CAD build for the part. Positions are in the model's coordinates, mm. A direction names the side the tool comes from. Give positions to 0.01 mm unless a question says otherwise; leave off trailing zeros. Order: outer loops, then holes, each group sorted by start corner. A loop starts at its lowest first (then second) coordinate and runs counter-clockwise, first axis right, second up.
```python
from build123d import *

# Parameters (mm, degrees)
SKETCH1_R               = 1.6
BOSS_EXTRUDE1_DEPTH     = 60
CUT_EXTRUDE1_DEPTH      = 165.822631941
SKETCH4_R               = 1.6
CUT_EXTRUDE2_DEPTH      = 165.822632055
CUT_EXTRUDE3_DEPTH      = 31.25
CUT_EXTRUDE3_DEPTH_BACK = 31.25
SKETCH5_W               = 5.6
SKETCH5_H               = 30
SKETCH8_R               = 1.6
CUT_EXTRUDE6_DEPTH      = 5
FILLET1_R               = 2
FILLET2_R               = 2
FILLET3_R               = 2
FILLET4_R               = 2
SKETCH9_W               = 7
SKETCH9_H               = 5.6
CUT_EXTRUDE7_DEPTH      = 3.5
SKETCH10_W              = 7
SKETCH10_H              = 5.6
CUT_EXTRUDE8_DEPTH      = 3.5


with BuildPart() as part:
    # Sketch1 → Boss-Extrude1 (new body)
    with BuildSketch(Plane(origin=(0, 0, 0), x_dir=(1, 0, 0), z_dir=(0, 1, 0))):
        with BuildLine():
            Line((0, 57.75), (0, 85.5))
            Line((0, 85.5), (127.5, 85.5))
            Line((127.5, 85.5), (127.5, 57.35))
            ThreePointArc((127.5, 57.35), (126.914213562, 55.935786438), (125.5, 55.35))
            Line((125.5, 55.35), (71.5, 55.35))
            ThreePointArc((71.5, 55.35), (69.9, 53.75), (71.5, 52.15))
            Line((71.5, 52.15), (125.5, 52.15))
            ThreePointArc((125.5, 52.15), (126.914213562, 51.564213562), (127.5, 50.15))
            Line((127.5, 50.15), (127.5, 35.35))
            ThreePointArc((127.5, 35.35), (126.914213562, 33.935786438), (125.5, 33.35))
            Line((125.5, 33.35), (71.5, 33.35))
            ThreePointArc((71.5, 33.35), (69.9, 31.75), (71.5, 30.15))
            Line((71.5, 30.15), (125.5, 30.15))
            ThreePointArc((125.5, 30.15), (126.914213562, 29.564213562), (127.5, 28.15))
            Line((127.5, 28.15), (127.5, 0))
            Line((127.5, 0), (0, 0))
            Line((0, 0), (0, 27.75))
            Line((0, 27.75), (0, 57.75))
        make_face()
        with Locations(Location((9.5, 53.75, 0), (0, 0, 270))):
            Circle(SKETCH1_R, mode=Mode.SUBTRACT)
        with Locations(Location((9.5, 31.75, 0), (0, 0, 270))):
            Circle(SKETCH1_R, mode=Mode.SUBTRACT)
        with BuildLine():
            Line((26.5, 15), (56.5, 15))
            ThreePointArc((56.5, 15), (63.571067812, 17.928932188), (66.5, 25))
            Line((66.5, 25), (66.5, 60.5))
            ThreePointArc((66.5, 60.5), (63.571067812, 67.571067812), (56.5, 70.5))
            Line((56.5, 70.5), (26.5, 70.5))
            ThreePointArc((26.5, 70.5), (19.428932188, 67.571067812), (16.5, 60.5))
            Line((16.5, 60.5), (16.5, 25))
            ThreePointArc((16.5, 25), (19.428932188, 17.928932188), (26.5, 15))
        make_face(mode=Mode.SUBTRACT)
    extrude(amount=BOSS_EXTRUDE1_DEPTH)

    # Sketch2 → Cut-Extrude1 (cut, through all)
    with BuildSketch(Plane.ZY):
        with BuildLine():
            Line((-70.5, 8), (-70.5, 3))
            Line((-70.5, 3), (-65.5, 3))
            Line((-65.5, 3), (-20, 3))
            Line((-20, 3), (-15, 3))
            Line((-15, 3), (-15, 8))
            Line((-15, 8), (-15, 49))
            ThreePointArc((-15, 49), (-16.464466094, 52.535533906), (-20, 54))
            Line((-20, 54), (-65.5, 54))
            ThreePointArc((-65.5, 54), (-69.035533906, 52.535533906), (-70.5, 49))
            Line((-70.5, 49), (-70.5, 8))
        make_face()
    extrude(amount=-CUT_EXTRUDE1_DEPTH, mode=Mode.SUBTRACT)

    # Sketch4 → Cut-Extrude2 (cut, through all)
    with BuildSketch(Plane(origin=(0, 0, -85.5), x_dir=(-1, 0, 0), z_dir=(0, 0, -1))):
        with Locations((-46, 55)):
            Circle(SKETCH4_R)
        with Locations((-31.5, 55)):
            Circle(SKETCH4_R)
        with BuildLine():
            Line((-56.25, 43.5), (-56.25, 13))
            ThreePointArc((-56.25, 13), (-54.785533906, 9.464466094), (-51.25, 8))
            Line((-51.25, 8), (-26.25, 8))
            ThreePointArc((-26.25, 8), (-22.714466094, 9.464466094), (-21.25, 13))
            Line((-21.25, 13), (-21.25, 43.5))
            ThreePointArc((-21.25, 43.5), (-22.714466094, 47.035533906), (-26.25, 48.5))
            Line((-26.25, 48.5), (-51.25, 48.5))
            ThreePointArc((-51.25, 48.5), (-54.785533906, 47.035533906), (-56.25, 43.5))
        make_face()
        with BuildLine():
            Line((-101.25, 48.5), (-76.25, 48.5))
            ThreePointArc((-76.25, 48.5), (-72.714466094, 47.035533906), (-71.25, 43.5))
            Line((-71.25, 43.5), (-71.25, 13))
            ThreePointArc((-71.25, 13), (-72.714466094, 9.464466094), (-76.25, 8))
            Line((-76.25, 8), (-101.25, 8))
            ThreePointArc((-101.25, 8), (-104.785533906, 9.464466094), (-106.25, 13))
            Line((-106.25, 13), (-106.25, 43.5))
            ThreePointArc((-106.25, 43.5), (-104.785533906, 47.035533906), (-101.25, 48.5))
        make_face()
        with BuildLine():
            Line((-112.85, 23.25), (-112.85, 48.25))
            ThreePointArc((-112.85, 48.25), (-111.25, 49.85), (-109.65, 48.25))
            Line((-109.65, 48.25), (-109.65, 23.25))
            ThreePointArc((-109.65, 23.25), (-111.25, 21.65), (-112.85, 23.25))
        make_face()
        with BuildLine():
            Line((-17.85, 23.25), (-17.85, 48.25))
            ThreePointArc((-17.85, 48.25), (-16.25, 49.85), (-14.65, 48.25))
            Line((-14.65, 48.25), (-14.65, 23.25))
            ThreePointArc((-14.65, 23.25), (-16.25, 21.65), (-17.85, 23.25))
        make_face()
    extrude(amount=-CUT_EXTRUDE2_DEPTH, mode=Mode.SUBTRACT)

    # Sketch5 → Cut-Extrude3 (cut, two sides: drawn at the far end of the back side and taken through both)
    with BuildSketch(Plane.XY.offset(-42.75).offset(-CUT_EXTRUDE3_DEPTH_BACK)):
        with Locations((16.25, 35.75)):
            Rectangle(SKETCH5_W, SKETCH5_H)
        with Locations((111.25, 35.75)):
            Rectangle(SKETCH5_W, SKETCH5_H)
    extrude(amount=CUT_EXTRUDE3_DEPTH + CUT_EXTRUDE3_DEPTH_BACK, mode=Mode.SUBTRACT)

    # SurfaceCut1
    split(bisect_by=Plane(origin=(0, 3, 0), x_dir=(1, 0, 0), z_dir=(0, 1, 0)), keep=Keep.TOP)

    # Sketch8 → Cut-Extrude6 (cut)
    with BuildSketch(Plane.XZ.offset(-3)):
        with Locations(Location((31.5, -7.5, 0), (0, 0, 270))):
            Circle(SKETCH8_R)
        with Locations(Location((46, -7.5, 0), (0, 0, 270))):
            Circle(SKETCH8_R)
        with Locations(Location((31.5, -78, 0), (0, 0, 270))):
            Circle(SKETCH8_R)
        with Locations(Location((46, -78, 0), (0, 0, 270))):
            Circle(SKETCH8_R)
        with Locations(Location((81.5, -7.5, 0), (0, 0, 270))):
            Circle(SKETCH8_R)
        with Locations(Location((96, -7.5, 0), (0, 0, 270))):
            Circle(SKETCH8_R)
        with Locations(Location((81.5, -78, 0), (0, 0, 270))):
            Circle(SKETCH8_R)
        with Locations(Location((96, -78, 0), (0, 0, 270))):
            Circle(SKETCH8_R)
    extrude(amount=-CUT_EXTRUDE6_DEPTH, mode=Mode.SUBTRACT)

    # Fillet1
    fillet1_edges = [part.edges().sort_by_distance(p)[0] for p in [
        (63.75, 3, 0),
    ]]
    fillet(fillet1_edges, radius=FILLET1_R)

    # Fillet2
    fillet2_edges = [part.edges().sort_by_distance(p)[0] for p in [
        (63.75, 3, -15),
    ]]
    fillet(fillet2_edges, radius=FILLET2_R)

    # Fillet3
    fillet3_edges = [part.edges().sort_by_distance(p)[0] for p in [
        (63.75, 3, -70.5),
    ]]
    fillet(fillet3_edges, radius=FILLET3_R)

    # Fillet4
    fillet4_edges = [part.edges().sort_by_distance(p)[0] for p in [
        (63.75, 3, -85.5),
    ]]
    fillet(fillet4_edges, radius=FILLET4_R)

    # Sketch9 → Cut-Extrude7 (cut)
    with BuildSketch(Plane(origin=(0, 0, -85.5), x_dir=(-1, 0, 0), z_dir=(0, 0, -1))):
        with Locations((-46, 55)):
            Rectangle(SKETCH9_W, SKETCH9_H)
        with Locations((-31.5, 55)):
            Rectangle(SKETCH9_W, SKETCH9_H)
    extrude(amount=-CUT_EXTRUDE7_DEPTH, mode=Mode.SUBTRACT)

    # Sketch10 → Cut-Extrude8 (cut)
    with BuildSketch(Plane.XY):
        with Locations((31.5, 55)):
            Rectangle(SKETCH10_W, SKETCH10_H)
        with Locations((46, 55)):
            Rectangle(SKETCH10_W, SKETCH10_H)
    extrude(amount=-CUT_EXTRUDE8_DEPTH, mode=Mode.SUBTRACT)


solid = part.part
```
Item 1: Slice it at A-A (z = -37). Give the cut face in (x, y).
Item 2: Slice it at B-B (x = 117). Give the cut face in (y, z), and give its area (3 significant figures).
Item 3: Tool access for faces 4 (the face through (99, 57, -55.35)), 5 (the face through (54.82, 9.5, -7.61)), 6 (the face through (31, 57.8, -2)), 7 (the face through (30.53, 5.46, -6.23)): list every direction of +Z, -Z, +X, -X, +Y, -Y with a clear straight run to the whole face (end or side of a thin tool).
Item 4: Drop flat-ended pins along their axis: pin 1 Ø10 at (x, y) = (51, 32.5) entering from -Z; pin 2 Ø5 at (x, y) = (31.5, 55) entering from +Z. Give the stop position or say it passes through.
Item 5: Slice it at D-D (z = -53.75). Give the cut face in (x, y), and give its area (3 significant figures).
Item 6: Wall check: L1, parallel to X at y = 12.5, z = -8.5; L2, parallel to X at y = 17.5, z = -76; L3, parallel to X at y = 6.65, z = -78. Give the ranges that are in metal, low to high.
Item 7: Slice it at C-C (y = 18). Give the cut face in (x, z).
Item 8: Two-plate mould, pull along Y, no slides. Class faces 1 (the face through (83.086, 5.465, -7.292)), 2 (the face through (91.5, 52.57, -69)), 3 (the face through (89, 48.5, -8)): released by +Y, released by -Y, zero draft, split by the parting line, or undercut.
A:
1. outline: (0, 54) - (16.5, 54) - (16.5, 60) - (0, 60) - close; (66.5, 54) - (127.5, 54) - (127.5, 60) - (66.5, 60) - close
2. outline: (3, -83.5) arc R2 ccw to (5, -85.5) - (60, -85.5) - (60, -55.35) - (54, -55.35) - (54, -65.5) arc R5 cw to (49, -70.5) - (5, -70.5) arc R2 ccw to (3, -72.5) - close; (3, -13) arc R2 ccw to (5, -15) - (49, -15) arc R5 cw to (54, -20) - (54, -30.15) - (60, -30.15) - (60, 0) - (5, 0) arc R2 ccw to (3, -2) - close; (54, -52.15) - (60, -52.15) - (60, -33.35) - (54, -33.35) - close
2. area: 2,010 mm2
3. face 4: +X, +Y, -Y
3. face 5: +Z, -Z
3. face 6: +Z
3. face 7: -Y
4. pin 1: passes through
4. pin 2: stops at z = -3.5
5. outline: (0, 54) - (7.9, 54) - (7.9, 60) - (0, 60) - close; (11.1, 54) - (16.5, 54) - (16.5, 60) - (11.1, 60) - close; (66.5, 54) - (69.9, 54) - (69.9, 60) - (66.5, 60) - close
5. area: 100 mm2
6. L1: x = 0 to 21.28, 56.22 to 71.28, 106.22 to 127.5
6. L2: x = 0 to 21.25, 56.25 to 71.25, 106.25 to 127.5
6. L3: x = 0 to 29.9, 33.1 to 44.4, 47.6 to 79.9, 83.1 to 94.4, 97.6 to 127.5
7. outline: (0, -85.5) - (21.25, -85.5) - (21.25, -70.5) - (0, -70.5) - close; (0, -15) - (21.25, -15) - (21.25, 0) - (0, 0) - close; (56.25, -85.5) - (71.25, -85.5) - (71.25, -70.5) - (56.25, -70.5) - close; (56.25, -15) - (71.25, -15) - (71.25, 0) - (56.25, 0) - close; (106.25, -85.5) - (127.5, -85.5) - (127.5, -70.5) - (106.25, -70.5) - close; (106.25, -15) - (127.5, -15) - (127.5, 0) - (106.25, 0) - close
8. face 1: zero draft
8. face 2: released by -Y
8. face 3: undercut
